CAD build for the part. Positions are in the model's coordinates, mm. A direction names the side the tool comes from. Coordinates: 2 decimals unless noted, no trailing zeros. Loops run counter-clockwise (first coordinate to the right, second up) from the corner with the lowest first, then second, coordinate; pieces in that order, holes last. Notation, with made-up numbers: (15.5, 25.5) -> (35.5, 25.5) arc R20 cw to (35.5, 57.5) -> close; hole circle Ø7 at (71, 13.25). An arc over 180 degrees is marked (long way). Write item = value, one per line. Start each with the question number.
(1) Band-saw the part on A-A (z = 111.76). Write the cut outline in (x, y).
(2) Flat gauge pins, fed straight in: P1, Ø10, axis at x = -29, z = 87.5, coming from the +Y side; P2, Ø3, axis at x = -12.7, y = -9.525, coming from the -Z side; P3, Ø5.5, axis at x = -33.5, y = -8, coming from the +Z side. Where does each tip first touch, or does it go through?
(3) Pull direction Y, two halves, no side cores. Call faces 1 (the face through (-25.4, -9, 102)), 2 (the face through (-12.88, -11.38, 108.2)), 3 (the face through (-26, 0, 50)): +Y half, -Y half, draft (parallel to the pull), parting line (faces both ways), or undercut.
(4) Tool access for faces 4 (the face through (0, -9, 63)), 5 (the face through (-15.06, -8.55, 12.88)), 6 (the face through (-44.45, -9, 101)): list every direction of +Z, -Z, +X, -X, +Y, -Y with a clear straight run to the whole face (end or side of a thin tool).
(5) Band-saw the part on C-C (x = -23). Write the cut outline in (y, z) (3 decimals), and give its area (3 significant figures).
(6) Drill centre lines: line 1 (X direction, y = -11.25, z = 88); line 2 (Y direction, x = -38, z = 11); line 3 (X direction, y = -7.25, z = 22). Where is each one in solid material? Low to high. Write a range as from..to.
(7) Band-saw the part on B-B (y = -1.25). Write the cut outline in (x, z), and give its area (3 significant figures).
```python
from build123d import *

# Parameters (mm, degrees)
F1_DEPTH = 19.05
F3_D     = 8.0264
F5_D     = 5.1054
F5_DEPTH = 25.4
F5_TIP   = 1.5338169022


with BuildPart() as f1:
    # F0 (on Front) → F1 (new body)
    with BuildSketch(Plane.XZ):
        Polygon((-50.8, 0), (0, 0), (0, 127), (-25.4, 127), (-25.4, 76.2), (-44.45, 76.2), (-44.45, 127), (-50.8, 127), align=None)
    extrude(amount=F1_DEPTH)

    # F3 (through all)
    with Locations(Plane.YZ):
        with Locations((-9.525, 111.76)):
            Hole(F3_D / 2)

    # F5
    with Locations(Plane(origin=(0, 0, 0), x_dir=(1, 0, 0), z_dir=(0, 0, -1))):
        with Locations((-38.1, 9.525), (-12.7, 9.525)):
            Hole(F5_D / 2, depth=F5_DEPTH)
            with Locations((0, 0, -(F5_DEPTH + F5_TIP / 2))):  # 118° drill point
                Cone(0, F5_D / 2, F5_TIP, mode=Mode.SUBTRACT)


solid = f1.part
```
Findings below:
q1.outline = (-50.8, -19.05) -> (-44.45, -19.05) -> (-44.45, -13.54) -> (-50.8, -13.54) -> close; (-50.8, -5.51) -> (-44.45, -5.51) -> (-44.45, 0) -> (-50.8, 0) -> close; (-25.4, -19.05) -> (0, -19.05) -> (0, -13.54) -> (-25.4, -13.54) -> close; (-25.4, -5.51) -> (0, -5.51) -> (0, 0) -> (-25.4, 0) -> close
q2.P1 = 0
q2.P2 = 26.03
q2.P3 = 76.2
q3.face_1 = draft
q3.face_2 = undercut
q3.face_3 = +Y half
q4.face_4 = +Z, -Z, +X, +Y, -Y
q4.face_5 = -Z
q4.face_6 = +Z, +Y, -Y
q5.outline = (-19.05, 0) -> (0, 0) -> (0, 127) -> (-19.05, 127) -> close; hole circle Ø8.026 at (-9.525, 111.76)
q5.area = 2,370 mm²
q6.line_1 = -50.8..-44.45, -25.4..0
q6.line_2 = -19.05..-12.08, -6.97..0
q6.line_3 = -50.8..-39.26, -36.94..-13.86, -11.54..0
q7.outline = (-50.8, 0) -> (0, 0) -> (0, 127) -> (-25.4, 127) -> (-25.4, 76.2) -> (-44.45, 76.2) -> (-44.45, 127) -> (-50.8, 127) -> close
q7.area = 5,480 mm²
